Read the model definition and answer for the solid it produces. Units are mm, in the model's axes. Face numbers are marked on the shaded views. A direction names the side the tool comes from. Coordinates: 2 decimals unless noted, no trailing zeros. Loops run counter-clockwise (first coordinate to the right, second up) from the corner with the lowest first, then second, coordinate; pieces in that order, holes last. Notation, with made-up numbers: (56.25, 41) - (85.25, 41) arc R9 ccw to (85.25, 55) - close; hole circle Ø2 at (-27.5, 71). An arc over 180 degrees is marked (long way). One line per item, written item: value. Start each with the question number.
from build123d import *

# Parameters (mm, degrees)
RESSALTO_EXTRUS_O1_DEPTH                    = 10
FURO_COM_FOLGA_DE_M61_D                     = 6.6
FURO_COM_FOLGA_DE_M61_DEPTH                 = 15
FURO_COM_FOLGA_DE_M61_TIP                   = 1.982840043
ESBO_O5_R                                   = 9.525
CORTE_EXTRUS_O1_DEPTH                       = 184.877003456
ESBO_O6_R                                   = 12.7
CORTE_EXTRUS_O2_DEPTH                       = 184.877003456
BROCA_DE_ROSQUEAR_PARA_TARRAXA_DE_M61_D     = 5
BROCA_DE_ROSQUEAR_PARA_TARRAXA_DE_M61_DEPTH = 15
BROCA_DE_ROSQUEAR_PARA_TARRAXA_DE_M61_TIP   = 1.502151548
BROCA_DE_ROSQUEAR_PARA_TARRAXA_DE_M62_D     = 5
BROCA_DE_ROSQUEAR_PARA_TARRAXA_DE_M62_DEPTH = 15
BROCA_DE_ROSQUEAR_PARA_TARRAXA_DE_M62_TIP   = 1.502151548
FURO_COM_FOLGA_DE_M81_D                     = 9
FURO_COM_FOLGA_DE_M51_D                     = 5.5
FURO_COM_FOLGA_DE_M51_DEPTH                 = 15
FURO_COM_FOLGA_DE_M51_TIP                   = 1.652366702
CORTE_EXTRUS_O5_DEPTH                       = 184.877003456
FURO_COM_FOLGA_DE_M62_D                     = 6.6
CORTE_EXTRUS_O6_DEPTH                       = 184.877003456
FILETE3_R                                   = 1.5


with BuildPart() as part:
    # Esboço2 → Ressalto-extrusão1 (new body)
    with BuildSketch(Plane(origin=(0, 0, 0), x_dir=(1, 0, 0), z_dir=(0, 1, 0))):
        Polygon((0, 0), (96.32, 0), (96.32, -5), (126.32, -5), (126.32, 0), (172.82, 0), (172.82, 57), (126.32, 57), (126.32, 62), (96.32, 62), (96.32, 57), (0, 57), align=None)
    extrude(amount=RESSALTO_EXTRUS_O1_DEPTH)

    # Furo com folga de M61
    with Locations(Plane(origin=(0, 10, 0), x_dir=(1, 0, 0), z_dir=(0, 1, 0))):
        with Locations((167.82, 46), (167.82, 28.5), (167.82, 11)):
            Hole(FURO_COM_FOLGA_DE_M61_D / 2, depth=FURO_COM_FOLGA_DE_M61_DEPTH)
            with Locations((0, 0, -(FURO_COM_FOLGA_DE_M61_DEPTH + FURO_COM_FOLGA_DE_M61_TIP / 2))):  # 118° drill point
                Cone(0, FURO_COM_FOLGA_DE_M61_D / 2, FURO_COM_FOLGA_DE_M61_TIP, mode=Mode.SUBTRACT)

    # Esboço5 → Corte-extrusão1 (cut, through all)
    with BuildSketch(Plane(origin=(0, 10, 0), x_dir=(1, 0, 0), z_dir=(0, 1, 0))):
        with Locations(Location((137.17, 28.5, 0), (0, 0, 270))):
            Circle(ESBO_O5_R)
    extrude(amount=-CORTE_EXTRUS_O1_DEPTH, mode=Mode.SUBTRACT)

    # Esboço6 → Corte-extrusão2 (cut, through all)
    with BuildSketch(Plane(origin=(0, 10, 0), x_dir=(1, 0, 0), z_dir=(0, 1, 0))):
        with Locations(Location((137.17, 28.5, 0), (0, 0, 270))):
            Circle(ESBO_O6_R)
    extrude(amount=-CORTE_EXTRUS_O2_DEPTH, mode=Mode.SUBTRACT)

    # Broca de rosquear para tarraxa de M61
    with Locations(Plane(origin=(0, 0, -57), x_dir=(-1, 0, 0), z_dir=(0, 0, -1))):
        with Locations((-148.17, 5), (-86.32, 5), (-71.32, 5)):
            Hole(BROCA_DE_ROSQUEAR_PARA_TARRAXA_DE_M61_D / 2, depth=BROCA_DE_ROSQUEAR_PARA_TARRAXA_DE_M61_DEPTH)
            with Locations((0, 0, -(BROCA_DE_ROSQUEAR_PARA_TARRAXA_DE_M61_DEPTH + BROCA_DE_ROSQUEAR_PARA_TARRAXA_DE_M61_TIP / 2))):  # 118° drill point
                Cone(0, BROCA_DE_ROSQUEAR_PARA_TARRAXA_DE_M61_D / 2, BROCA_DE_ROSQUEAR_PARA_TARRAXA_DE_M61_TIP, mode=Mode.SUBTRACT)

    # Broca de rosquear para tarraxa de M62
    with Locations(Plane.XY):
        with Locations((86.32, 5), (148.17, 5), (71.32, 5)):
            Hole(BROCA_DE_ROSQUEAR_PARA_TARRAXA_DE_M62_D / 2, depth=BROCA_DE_ROSQUEAR_PARA_TARRAXA_DE_M62_DEPTH)
            with Locations((0, 0, -(BROCA_DE_ROSQUEAR_PARA_TARRAXA_DE_M62_DEPTH + BROCA_DE_ROSQUEAR_PARA_TARRAXA_DE_M62_TIP / 2))):  # 118° drill point
                Cone(0, BROCA_DE_ROSQUEAR_PARA_TARRAXA_DE_M62_D / 2, BROCA_DE_ROSQUEAR_PARA_TARRAXA_DE_M62_TIP, mode=Mode.SUBTRACT)

    # Furo com folga de M81 (through all)
    with Locations(Plane(origin=(0, 10, 0), x_dir=(1, 0, 0), z_dir=(0, 1, 0))):
        with Locations((42, 46), (42, 28.5), (42, 11)):
            Hole(FURO_COM_FOLGA_DE_M81_D / 2)

    # Furo com folga de M51
    with Locations(Plane(origin=(0, 10, 0), x_dir=(1, 0, 0), z_dir=(0, 1, 0))):
        with Locations((156.64, 51.5), (156.64, 5.5), (60, 5.5), (60, 51.5)):
            Hole(FURO_COM_FOLGA_DE_M51_D / 2, depth=FURO_COM_FOLGA_DE_M51_DEPTH)
            with Locations((0, 0, -(FURO_COM_FOLGA_DE_M51_DEPTH + FURO_COM_FOLGA_DE_M51_TIP / 2))):  # 118° drill point
                Cone(0, FURO_COM_FOLGA_DE_M51_D / 2, FURO_COM_FOLGA_DE_M51_TIP, mode=Mode.SUBTRACT)

    # Esboço22 → Corte-extrusão5 (cut, through all)
    with BuildSketch(Plane(origin=(0, 10, 0), x_dir=(1, 0, 0), z_dir=(0, 1, 0))):
        Polygon((0, 0), (0, 57), (15.273103969, 57), align=None)
    extrude(amount=-CORTE_EXTRUS_O5_DEPTH, mode=Mode.SUBTRACT)

    # Furo com folga de M62 (through all)
    with Locations(Plane(origin=(0, 0, 0), x_dir=(-1, 0, 0), z_dir=(0, -1, 0))):
        with Locations((-22.851404532, 40), (-15.086833179, 11.022225211), (-18.969118855, 25.511112606)):
            Hole(FURO_COM_FOLGA_DE_M62_D / 2)

    # Esboço25 → Corte-extrusão6 (cut, through all)
    with BuildSketch(Plane(origin=(0, 10, 0), x_dir=(1, 0, 0), z_dir=(0, 1, 0))):
        Polygon((64.82, 9), (50.82, 28.5), (64.82, 48), align=None)
        Polygon((93.82, 51), (111.241406328, 51), (93.82, 6), align=None)
        Polygon((102.398593672, 6), (119.82, 51), (119.82, 6), align=None)
    extrude(amount=-CORTE_EXTRUS_O6_DEPTH, mode=Mode.SUBTRACT)

    # Filete3
    filete3_edges = [part.edges().sort_by_distance(p)[0] for p in [
        (64.82, 5, -48),
        (64.82, 5, -9),
        (50.82, 5, -28.5),
        (119.82, 5, -6),
        (102.398593672, 5, -6),
        (119.82, 5, -51),
        (93.82, 5, -6),
        (93.82, 5, -51),
        (111.241406328, 5, -51),
    ]]
    fillet(filete3_edges, radius=FILETE3_R)


solid = part.part
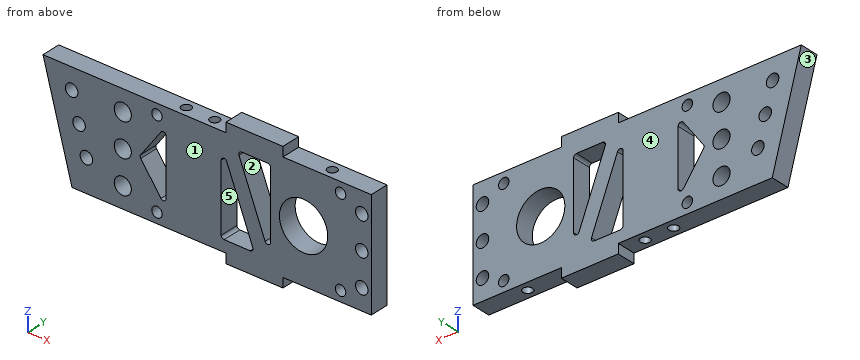
1) Section C-C, the plane x = 156.64 is taken. Determine the outline of the cut face in (y, z).
2) For the marked faces 1 and 2, determine the directions among +Z, -Z, +X, -X, +Y, -Y from which every point of the face is accessible in a straight line to the end or side of a thin tool.
3) Section B-B, the plane x = 42 is taken. Determine the outline of the cut face in (y, z), and give its area (3 significant figures).
4) Flat-ended cylindrical pins translate along their axes: P1, Ø1.5, axis at x = 86.5, z = -55, coming from the -Y side; P2, Ø5, axis at x = 75, y = 6.5, coming from the -Z side; P3, Ø3, axis at y = 2.5, z = -3, coming from the -X side; P4, Ø4, axis at y = 3.5, z = -43, coming from the -X side. Find the tip coordinate at first contact, or state that the pin passes through.
5) Straight lines are drawn through the part: L1, parallel to Z at x = 167.82, y = 2.5; L2, parallel to Z at x = 60, y = 6.25; L3, parallel to X at y = 5, z = -54. For each, find the intervals that lie inside material, in ascending order.
6) Determine the mould class of the marked faces 3, 4 and 5 for opening direction Z: released by +Z, released by -Z, zero draft, split by the parting line, or undercut.
7) Section A-A, the plane x = 137.17 is taken. Determine the outline of the cut face in (y, z), and give its area (3 significant figures).
Answer below:
1. outline: (0, -57) - (10, -57) - (10, -54.25) - (0, -54.25) - close; (0, -48.75) - (10, -48.75) - (10, -8.25) - (0, -8.25) - close; (0, -2.75) - (10, -2.75) - (10, 0) - (0, 0) - close
2. face 1: +Z, -Z, +X, -X, -Y
2. face 2: +Y, -Y
3. outline: (0, -57) - (10, -57) - (10, -50.5) - (0, -50.5) - close; (0, -41.5) - (10, -41.5) - (10, -33) - (0, -33) - close; (0, -24) - (10, -24) - (10, -15.5) - (0, -15.5) - close; (0, -6.5) - (10, -6.5) - (10, 0) - (0, 0) - close
3. area: 300 mm2
4. P1: y = 0
4. P2: z = -57
4. P3: x = 0.4
4. P4: x = 10.99
5. L1: -57 to -49.3, -42.7 to -31.8, -25.2 to -14.3, -7.7 to 0
5. L2: -57 to -54.25, -48.75 to -41.29, -15.71 to -8.25, -2.75 to 0
5. L3: 14.47 to 58.85, 61.15 to 68.82, 73.82 to 83.82, 88.82 to 145.67, 150.67 to 155.49, 157.79 to 172.82
6. face 3: released by -Z
6. face 4: zero draft
6. face 5: undercut
7. outline: (0, -57) - (10, -57) - (10, -41.2) - (0, -41.2) - close; (0, -15.8) - (10, -15.8) - (10, 0) - (0, 0) - close
7. area: 316 mm2
